```python
from build123d import *

# Parameters (mm, degrees)
SKETCH_2_R          = 2.55
EXTRUDE_1_DEPTH     = 100
SKETCH_3_R          = 3
CUT_EXTRUDE_1_DEPTH = 103.46950766


with BuildPart() as part:
    # 草图2 → 凸台-拉伸1 (new body)
    with BuildSketch(Plane.XY):
        with BuildLine():
            Line((-3.9, 2.839339828), (-6.560660172, 5.5))
            Line((-6.560660172, 5.5), (-8.2, 5.5))
            Line((-8.2, 5.5), (-8.2, 3.1))
            Line((-8.2, 3.1), (-9.45, 3.1))
            Line((-9.45, 3.1), (-9.45, 3.65))
            Line((-9.45, 3.65), (-10, 3.65))
            Line((-10, 3.65), (-10, 8.5))
            ThreePointArc((-10, 8.5), (-9.560660172, 9.560660172), (-8.5, 10))
            Line((-8.5, 10), (-3.65, 10))
            Line((-3.65, 10), (-3.65, 9.45))
            Line((-3.65, 9.45), (-3.1, 9.45))
            Line((-3.1, 9.45), (-3.1, 8.2))
            Line((-3.1, 8.2), (-5.5, 8.2))
            Line((-5.5, 8.2), (-5.5, 6.560660172))
            Line((-5.5, 6.560660172), (-2.839339828, 3.9))
            Line((-2.839339828, 3.9), (2.839339828, 3.9))
            Line((2.839339828, 3.9), (5.5, 6.560660172))
            Line((5.5, 6.560660172), (5.5, 8.2))
            Line((5.5, 8.2), (3.1, 8.2))
            Line((3.1, 8.2), (3.1, 9.45))
            Line((3.1, 9.45), (3.65, 9.45))
            Line((3.65, 9.45), (3.65, 10))
            Line((3.65, 10), (8.5, 10))
            ThreePointArc((8.5, 10), (9.560660172, 9.560660172), (10, 8.5))
            Line((10, 8.5), (10, 3.65))
            Line((10, 3.65), (9.45, 3.65))
            Line((9.45, 3.65), (9.45, 3.1))
            Line((9.45, 3.1), (8.2, 3.1))
            Line((8.2, 3.1), (8.2, 5.5))
            Line((8.2, 5.5), (6.560660172, 5.5))
            Line((6.560660172, 5.5), (3.9, 2.839339828))
            Line((3.9, 2.839339828), (3.9, -2.839339828))
            Line((3.9, -2.839339828), (6.560660172, -5.5))
            Line((6.560660172, -5.5), (8.2, -5.5))
            Line((8.2, -5.5), (8.2, -3.1))
            Line((8.2, -3.1), (9.45, -3.1))
            Line((9.45, -3.1), (9.45, -3.65))
            Line((9.45, -3.65), (10, -3.65))
            Line((10, -3.65), (10, -8.5))
            ThreePointArc((10, -8.5), (9.560660172, -9.560660172), (8.5, -10))
            Line((8.5, -10), (3.65, -10))
            Line((3.65, -10), (3.65, -9.45))
            Line((3.65, -9.45), (3.1, -9.45))
            Line((3.1, -9.45), (3.1, -8.2))
            Line((3.1, -8.2), (5.5, -8.2))
            Line((5.5, -8.2), (5.5, -6.560660172))
            Line((5.5, -6.560660172), (2.839339828, -3.9))
            Line((2.839339828, -3.9), (-2.839339828, -3.9))
            Line((-2.839339828, -3.9), (-5.5, -6.560660172))
            Line((-5.5, -6.560660172), (-5.5, -8.2))
            Line((-5.5, -8.2), (-3.1, -8.2))
            Line((-3.1, -8.2), (-3.1, -9.45))
            Line((-3.1, -9.45), (-3.65, -9.45))
            Line((-3.65, -9.45), (-3.65, -10))
            Line((-3.65, -10), (-8.5, -10))
            ThreePointArc((-8.5, -10), (-9.560660172, -9.560660172), (-10, -8.5))
            Line((-10, -8.5), (-10, -3.65))
            Line((-10, -3.65), (-9.45, -3.65))
            Line((-9.45, -3.65), (-9.45, -3.1))
            Line((-9.45, -3.1), (-8.2, -3.1))
            Line((-8.2, -3.1), (-8.2, -5.5))
            Line((-8.2, -5.5), (-6.560660172, -5.5))
            Line((-6.560660172, -5.5), (-3.9, -2.839339828))
            Line((-3.9, -2.839339828), (-3.9, 2.839339828))
        make_face()
        Circle(SKETCH_2_R, mode=Mode.SUBTRACT)
    extrude(amount=EXTRUDE_1_DEPTH)

    # 草图3 → 切除-拉伸1 (cut, through all)
    with BuildSketch(Plane(origin=(10, 0, 0), x_dir=(0, 0, -1), z_dir=(1, 0, 0))):
        with Locations(Location((-90, 0, 0), (0, 0, 108.835996158))):
            Circle(SKETCH_3_R)
        with Locations(Location((-10, 0, 0), (0, 0, 108.835996158))):
            Circle(SKETCH_3_R)
    extrude(amount=-CUT_EXTRUDE_1_DEPTH, mode=Mode.SUBTRACT)


solid = part.part
```
Model file for the job. Use its own axes, mm. A direction names the side the tool comes from. Coordinates: 2 decimals unless noted, no trailing zeros. Loops run counter-clockwise (first coordinate to the right, second up) from the corner with the lowest first, then second, coordinate; pieces in that order, holes last. Notation, with made-up numbers: M -21.75,-34.5 L 30.25,-34.5 A34 cw 30.25,-1.5 Z; hole C 55.25,-32.75 d8. An arc over 180 degrees is marked long. Use CSV: the item, a comma, the result in double quotes. Start each with the question number.
1. Band-saw the part on B-B, the plane y = 0. List the corners of the cut face in (x, z), then the cut area to 3 significant figures.
2. Band-saw the part on A-A, the plane x = 0. List the corners of the cut face in (y, z), then the cut area to 3 significant figures.
3. Tool access for faces 1 (the flat face through (3.9, 0, 49)), 2 (the flat face through (-3.9, 0, 3)), 3 (the flat face through (-8.2, 4, 49)), 4 (the flat face through (6, -10, 49)): list every direction of +Z, -Z, +X, -X, +Y, -Y with a clear straight run to the whole face (end or side of a thin tool).
4. Two-plate mould, pull along X, no slides. Class faces 5 (the flat face through (0, -3.9, 49)), 6 (the flat face through (3.9, 0, 96)), 7 (the flat face through (-3.9, 0, 96)): pulls with the +X half, pulls with the -X half, needs draft (parallel to the pull), parting line crosses it, or undercut.
5. Probe probe 1 along Y at (x, z) = (-0.25, 90); probe 2 along X at (y, z) = (0, 5.75); probe 3 along X at (y, z) = (7, 43.5). List the from-to ranges inside material, lowest first. Write a range as [from, to].
6. Flat gauge pins, fed straight in: pin 1 (7 mm diameter, centred on y = 0, z = 90, fed in from -X); pin 2 (0.6 mm diameter, centred on x = 9, z = 27, fed in from -Y); pin 3 (2 mm diameter, centred on x = 1, z = 66, fed in from +Y). Where does each tip first touch, or does it go through?
Entries:
1,outline,"M -3.9,0 L -2.55,0 L -2.55,7 L -3.9,7 Z; M -3.9,13 L -2.55,13 L -2.55,87 L -3.9,87 Z; M -3.9,93 L -2.55,93 L -2.55,100 L -3.9,100 Z; M 2.55,0 L 3.9,0 L 3.9,7 L 2.55,7 Z; M 2.55,13 L 3.9,13 L 3.9,87 L 2.55,87 Z; M 2.55,93 L 3.9,93 L 3.9,100 L 2.55,100 Z"
1,area,"238 mm2"
2,outline,"M -3.9,0 L -2.55,0 L -2.55,8.42 A3 cw -2.55,11.58 L -2.55,88.42 A3 cw -2.55,91.58 L -2.55,100 L -3.9,100 Z; M 2.55,0 L 3.9,0 L 3.9,100 L 2.55,100 L 2.55,91.58 A3 cw 2.55,88.42 L 2.55,11.58 A3 cw 2.55,8.42 Z"
2,area,"266 mm2"
3,face 1,"+Z, -Z, +X"
3,face 2,"+Z, -Z, -X"
3,face 3,"+Z, -Z"
3,face 4,"+Z, -Z, +X, -X, -Y"
4,face 5,"undercut"
4,face 6,"pulls with the +X half"
4,face 7,"pulls with the -X half"
5,probe 1,"y = [-3.9, -3], [3, 3.9]"
5,probe 2,"x = [-3.9, -2.55], [2.55, 3.9]"
5,probe 3,"x = [-10, -5.5], [5.5, 10]"
6,pin 1,"stops at x = -9.45"
6,pin 2,"stops at y = -9.99"
6,pin 3,"stops at y = 3.9"
